```python
from build123d import *

# Parameters (mm, degrees)
ESBO_O4_R                = 1.65
RESSALTO_EXTRUS_O2_DEPTH = 2
ESBO_O5_R                = 14
RESSALTO_EXTRUS_O3_DEPTH = 20
ESBO_O6_R                = 13.2
CORTE_EXTRUS_O1_DEPTH    = 20


with BuildPart() as part:
    # Esboço4 → Ressalto-extrusão2 (new body)
    with BuildSketch(Plane(origin=(0, 0, 0), x_dir=(1, 0, 0), z_dir=(0, 1, 0))):
        with BuildLine():
            Line((-19.257073584, -4.5), (-13.257073584, -4.5))
            ThreePointArc((-13.257073584, -4.5), (-7, -12.124355653), (2.731422475, -13.730962503))
            Line((2.731422475, -13.730962503), (5.731422475, -18.927114926))
            ThreePointArc((5.731422475, -18.927114926), (10.832700248, -18.762787213), (13.525651109, -14.427114926))
            Line((13.525651109, -14.427114926), (10.525651109, -9.230962503))
            ThreePointArc((10.525651109, -9.230962503), (14, 0), (10.525651109, 9.230962503))
            Line((10.525651109, 9.230962503), (13.525651109, 14.427114926))
            ThreePointArc((13.525651109, 14.427114926), (10.832700248, 18.762787213), (5.731422475, 18.927114926))
            Line((5.731422475, 18.927114926), (2.731422475, 13.730962503))
            ThreePointArc((2.731422475, 13.730962503), (-7, 12.124355653), (-13.257073584, 4.5))
            Line((-13.257073584, 4.5), (-19.257073584, 4.5))
            ThreePointArc((-19.257073584, 4.5), (-21.665400497, 0), (-19.257073584, -4.5))
        make_face()
        with Locations(Location((-19, 0, 0), (0, 0, 270))):
            Circle(ESBO_O4_R, mode=Mode.SUBTRACT)
        with Locations(Location((9.5, 16.454482672, 0), (0, 0, 270))):
            Circle(ESBO_O4_R, mode=Mode.SUBTRACT)
        with Locations(Location((9.5, -16.454482672, 0), (0, 0, 270))):
            Circle(ESBO_O4_R, mode=Mode.SUBTRACT)
    extrude(amount=RESSALTO_EXTRUS_O2_DEPTH)

    # Esboço5 → Ressalto-extrusão3 (add)
    with BuildSketch(Plane(origin=(0, 2, 0), x_dir=(1, 0, 0), z_dir=(0, 1, 0))):
        with Locations(Location((0, 0, 0), (0, 0, 78.749340847))):
            Circle(ESBO_O5_R)
    extrude(amount=RESSALTO_EXTRUS_O3_DEPTH)

    # Esboço6 → Corte-extrusão1 (cut)
    with BuildSketch(Plane(origin=(0, 22, 0), x_dir=(1, 0, 0), z_dir=(0, 1, 0))):
        with Locations(Location((0, 0, 0), (0, 0, 270))):
            Circle(ESBO_O6_R)
    extrude(amount=-CORTE_EXTRUS_O1_DEPTH, mode=Mode.SUBTRACT)


solid = part.part
```
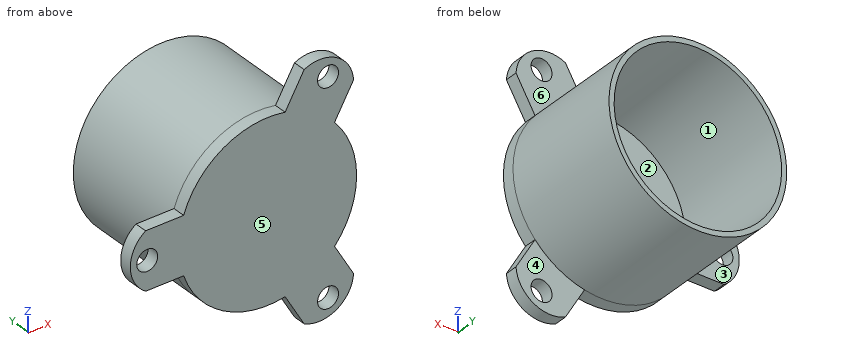
Verification items for the finished model (mm, model axes). Face numbers are marked on the shaded views. A direction names the side the tool comes from. Coordinates: 2 decimals unless noted, no trailing zeros. Write each loop counter-clockwise with the first axis right and the second up, starting at its lowest first coordinate (ties: lowest second). Pieces come first, ordered by that corner, then holes. Notation, with made-up numbers: M -20.75,54 L -7.75,54 A19 cw -7.75,61 Z; hole C 58.5,34.5 d5. An arc over 180 degrees is marked long. Answer as a JSON object with one key per item and string values. Group by question number.
(1) Cross-section at D-D, the plane x = 0. Record the cut outline in (y, z).
(2) Gauge pin test, flat ends, axial feed: pin 1 (16 mm diameter, centred on x = 0, z = 0, fed in from +Y); pin 2 (8 mm diameter, centred on x = -13, y = 9, fed in from -Z); pin 3 (2 mm diameter, centred on y = 7, z = 3, fed in from -X); pin 4 (3 mm diameter, centred on x = -16.5, y = 13.5, fed in from -Z). Record the tip position at first contact, or that the pin passes through.
(3) Cross-section at C-C, the plane y = 18. Record the cut outline in (x, z).
(4) Material ranges on line 1 (X direction, y = 4.75, z = 0.5); line 2 (Z direction, x = -5, y = 18.5); line 3 (Z direction, x = 10, y = 12.75), recorded low to high.
(5) Release check for a two-part mould opening along X. For the marked faces 1, 2 and 3 record: +X half, -X half, draft (parallel to the pull), parting line (faces both ways), or undercut.
(6) Cross-section at A-A, the plane z = 0. Record the cut outline in (x, y), and give its area (3 significant figures).
(7) Tool access check on the marked faces 4, 5 and 6. Record the directions out of +Z, -Z, +X, -X, +Y, -Y that give a thin tool (end or side, any length) a straight path to the whole face; none if there is none.
(8) Cross-section at B-B, the plane x = 9. Record the cut outline in (y, z).
Reply:
{
 "1": {"outline": "M 0,-14 L 22,-14 L 22,-13.2 L 2,-13.2 L 2,13.2 L 22,13.2 L 22,14 L 0,14 Z"},
 "2": {"pin 1": "y = 2", "pin 2": "z = -10.72", "pin 3": "x = -13.86", "pin 4": "through"},
 "3": {"outline": "C 0,0 d28; hole C 0,0 d26.4"},
 "4": {"line 1": "-13.99 to -13.19, 13.19 to 13.99", "line 2": "-13.08 to -12.22, 12.22 to 13.08", "line 3": "-9.8 to -8.62, 8.62 to 9.8"},
 "5": {"face 1": "undercut", "face 2": "undercut", "face 3": "draft"},
 "6": {"outline": "M -21.67,0 L -20.65,0 L -20.65,2 L -21.67,2 Z; M -17.35,0 L 14,0 L 14,22 L 13.2,22 L 13.2,2 L -13.2,2 L -13.2,22 L -14,22 L -14,2 L -17.35,2 Z", "area": "96.7 mm²"},
 "7": {"face 4": "-Z, +X, +Y", "face 5": "+Z, -Z, +X, -X, -Y", "face 6": "+Z, +X, +Y"},
 "8": {"outline": "M 0,-19.42 L 2,-19.42 L 2,-18.03 L 0,-18.03 Z; M 0,-14.88 L 2,-14.88 L 2,-10.72 L 22,-10.72 L 22,-9.66 L 2,-9.66 L 2,9.66 L 22,9.66 L 22,10.72 L 2,10.72 L 2,14.88 L 0,14.88 Z; M 0,18.03 L 2,18.03 L 2,19.42 L 0,19.42 Z"}
}
